Could you check a few things on this model? Use its own coordinates, in mm. A direction names the side the tool comes from. Give positions to 0.01 mm unless a question says otherwise; leave off trailing zeros. Loops run counter-clockwise (first coordinate to the right, second up) from the corner with the lowest first, then second, coordinate; pieces in that order, holes last. Notation, with made-up numbers: (-28, -16) - (1, -16) arc R16 cw to (1, -3) - close; hole circle Ø2 at (-22.75, -33). An arc over 180 degrees is marked (long way). Write each question's results on one line, items separated by ' | '. Start each with the question number.
1) On a 3-axis mill with a long thin cutter (end or side, diameter ignored), from which of +Z, -Z, +X, -X, +Y, -Y can I reach the whole of each face in a straight line? I mean faces 1 (the face through (6.35, 2, 3)), 2 (the face through (106.35, 2, -100)), 3 (the face through (56, 9, -87.63)). Say none if no direction works.
2) I want a section at B-B, the plane x = 29.5. Write out the boundary of the cut face in (y, z), and give its area (3 significant figures).
3) I'm going to push flat-ended pins straight in: pin 1 (4 mm diameter, centred on x = 3.175, z = -99.695, fed in from +Y) (3 decimals); pin 2 (3 mm diameter, centred on x = 73, z = -52, fed in from +Y); pin 3 (1.5 mm diameter, centred on y = 9.5, z = -80.5, fed in from +X); pin 4 (1.9 mm diameter, centred on x = 63, y = 6, fed in from +Z). Where does each tip first touch, or does it pass through?
4) If I drill on probe 1 along Z at (x, y) = (65.5, 5.75); probe 2 along X at (y, z) = (4, -33.5); probe 3 along Y at (x, z) = (52, -88), over which ranges is the centre line in solid material (lowest first)? Write a range as [from, to].
5) If we mould it in two halves opening along Y, with no side actions, what happens to faces 4 (the face through (56, 7.62, -91)), 5 (the face through (5, 3.175, 2)), 6 (the face through (56, 6, -96.52))? For each: +Y half, -Y half, draft (parallel to the pull), parting line (faces both ways), or undercut.
6) I want a section at C-C, the plane z = -34.5. Write out the boundary of the cut face in (x, y), and give its area (3 significant figures).
7) I want a section at A-A, the plane y = 5.5. Write out the boundary of the cut face in (x, z), and give its area (3 significant figures).
from build123d import *

# Parameters (mm, degrees)
SKETCH1_W           = 112.699999898
SKETCH1_H           = 96.52
BOSS_EXTRUDE1_DEPTH = 7.62
SKETCH2_W           = 104.14
SKETCH2_H           = 91.44
CUT_EXTRUDE1_DEPTH  = 3.81
SKETCH3_W           = 6.35
SKETCH3_H           = 6.35
SKETCH3_R           = 1.7
BOSS_EXTRUDE2_DEPTH = 3.175
SKETCH4_W           = 112.699999898
SKETCH4_H           = 8.89
BOSS_EXTRUDE3_DEPTH = 3.81


with BuildPart() as part:
    # Sketch1 → Boss-Extrude1 (new body)
    with BuildSketch(Plane(origin=(0, 0, 0), x_dir=(1, 0, 0), z_dir=(0, 1, 0))):
        with Locations((56.349999949, 48.26)):
            Rectangle(SKETCH1_W, SKETCH1_H)
    extrude(amount=BOSS_EXTRUDE1_DEPTH)

    # Sketch2 → Cut-Extrude1 (cut)
    with BuildSketch(Plane(origin=(0, 7.62, 0), x_dir=(1, 0, 0), z_dir=(0, 1, 0))):
        with Locations((56.349999949, 48.26)):
            Rectangle(SKETCH2_W, SKETCH2_H)
    extrude(amount=-CUT_EXTRUDE1_DEPTH, mode=Mode.SUBTRACT)

    # Sketch3 → Boss-Extrude2 (add)
    # profile 1 of 4: a face of its own
    with BuildSketch(Plane.XZ):
        with Locations((109.524999898, 3.175)):
            Rectangle(SKETCH3_W, SKETCH3_H)
        with Locations(Location((109.524999898, 3.175, 0), (0, 0, 270))):
            Circle(SKETCH3_R, mode=Mode.SUBTRACT)
    # profile 2 of 4: a face of its own
    with BuildSketch(Plane.XZ):
        with Locations((3.175, 3.175)):
            Rectangle(SKETCH3_W, SKETCH3_H)
        with Locations(Location((3.175, 3.175, 0), (0, 0, 270))):
            Circle(SKETCH3_R, mode=Mode.SUBTRACT)
    # profile 3 of 4: a face of its own
    with BuildSketch(Plane.XZ):
        with Locations((3.175, -99.695)):
            Rectangle(SKETCH3_W, SKETCH3_H)
        with Locations(Location((3.175, -99.695, 0), (0, 0, 270))):
            Circle(SKETCH3_R, mode=Mode.SUBTRACT)
    # profile 4 of 4: a face of its own
    with BuildSketch(Plane.XZ):
        with Locations((109.524999898, -99.695)):
            Rectangle(SKETCH3_W, SKETCH3_H)
        with Locations(Location((109.524999898, -99.695, 0), (0, 0, 270))):
            Circle(SKETCH3_R, mode=Mode.SUBTRACT)
    extrude(amount=-BOSS_EXTRUDE2_DEPTH)

    # Sketch4 → Boss-Extrude3 (add)
    with BuildSketch(Plane(origin=(0, 7.62, 0), x_dir=(1, 0, 0), z_dir=(0, 1, 0))):
        with Locations((56.349999949, 92.075)):
            Rectangle(SKETCH4_W, SKETCH4_H)
    extrude(amount=BOSS_EXTRUDE3_DEPTH)


solid = part.part
Answers:
1) face 1: +Z, +Y, -Y | face 2: -Z, +Y, -Y | face 3: +Z, +X, -X, +Y
2) outline: (0, -96.52) - (11.43, -96.52) - (11.43, -87.63) - (7.62, -87.63) - (7.62, -93.98) - (3.81, -93.98) - (3.81, -2.54) - (7.62, -2.54) - (7.62, 0) - (0, 0) - close | area: 421 mm2
3) pin 1: stops at y = 3.175 | pin 2: stops at y = 3.81 | pin 3: passes through | pin 4: stops at z = 0
4) probe 1: z = [-96.52, -93.98], [-2.54, 0] | probe 2: x = [0, 4.28], [108.42, 112.7] | probe 3: y = [0, 3.81], [7.62, 11.43]
5) face 4: undercut | face 5: +Y half | face 6: draft
6) outline: (0, 0) - (112.7, 0) - (112.7, 7.62) - (108.42, 7.62) - (108.42, 3.81) - (4.28, 3.81) - (4.28, 7.62) - (0, 7.62) - close | area: 462 mm2
7) outline: (0, -96.52) - (112.7, -96.52) - (112.7, 0) - (0, 0) - close; hole (4.28, -93.98) - (108.42, -93.98) - (108.42, -2.54) - (4.28, -2.54) - close | area: 1,360 mm2
